CAD build for the part. Positions are in the model's coordinates, mm. A direction names the side the tool comes from. Round coordinates to 2 decimals unless told otherwise and drop trailing zeros. Order: outer loops, then holes, each group sorted by start corner. A loop starts at its lowest first (then second) coordinate and runs counter-clockwise, first axis right, second up. Notation, with made-up numbers: (81.5, 80.5) - (107.5, 80.5) arc R7 ccw to (107.5, 91.5) - close; hole circle Ø1 at (-35.75, 0.5). An arc over 180 degrees is marked (long way). Use one line per item in the form item = value. Start each with the question number.
from build123d import *

# Parameters (mm, degrees)
SKETCH1_W           = 60.96
SKETCH1_H           = 40.64
BOSS_EXTRUDE1_DEPTH = 5.08
SHELL1_T            = -2.54
SKETCH2_R           = 2.54
BOSS_EXTRUDE2_DEPTH = 5.08
SKETCH3_R           = 1.016
CUT_EXTRUDE1_DEPTH  = 5.08
FILLET2_R           = 1.27


with BuildPart() as part:
    # Sketch1 → Boss-Extrude1 (new body)
    with BuildSketch(Plane(origin=(0, 0, 0), x_dir=(1, 0, 0), z_dir=(0, 1, 0))):
        with Locations((30.48, 20.32)):
            Rectangle(SKETCH1_W, SKETCH1_H)
    extrude(amount=BOSS_EXTRUDE1_DEPTH)

    # Shell1
    shell1_openings = [part.faces().sort_by_distance(p)[0] for p in [
        (30.48, 0, -20.32),
    ]]
    offset(amount=SHELL1_T, openings=shell1_openings, kind=Kind.INTERSECTION)

    # Sketch2 → Boss-Extrude2 (add)
    with BuildSketch(Plane.XZ):
        with Locations((58.42, -38.1)):
            Circle(SKETCH2_R)
        with Locations((58.42, -2.54)):
            Circle(SKETCH2_R)
        with Locations((2.54, -2.54)):
            Circle(SKETCH2_R)
        with Locations((2.54, -38.1)):
            Circle(SKETCH2_R)
    extrude(amount=-BOSS_EXTRUDE2_DEPTH)

    # Sketch3 → Cut-Extrude1 (cut)
    with BuildSketch(Plane.XZ):
        with Locations((58.42, -38.1)):
            Circle(SKETCH3_R)
        with Locations((58.42, -2.54)):
            Circle(SKETCH3_R)
        with Locations((2.54, -2.54)):
            Circle(SKETCH3_R)
        with Locations((2.54, -38.1)):
            Circle(SKETCH3_R)
    extrude(amount=-CUT_EXTRUDE1_DEPTH, mode=Mode.SUBTRACT)

    # Fillet2
    fillet2_edges = [part.edges().sort_by_distance(p)[0] for p in [
        (60.96, 5.08, -20.32),
        (30.48, 5.08, -40.64),
        (0, 5.08, -20.32),
        (30.48, 5.08, 0),
        (0, 2.54, -40.64),
        (60.96, 2.54, -40.64),
        (60.96, 2.54, 0),
        (0, 2.54, 0),
    ]]
    fillet(fillet2_edges, radius=FILLET2_R)


solid = part.part
(1) Mould opens along X. For faces 1 (the flat face through (30, 2.54, -21)), 2 (the cylindrical face through (0.382, 4.718, -20.053)), 3 (the cylindrical face through (30.071, 4.718, -40.258)) say: pulls with the +X half, pulls with the -X half, needs draft (parallel to the pull), parting line crosses it, or undercut.
(2) Slice it at B-B (y = 1.5). Give the cut face in (x, z).
(3) Slice it at A-A (z = -6). Give the cut face in (x, y), and give its area (3 significant figures).
(4) Flat gauge pins, fed straight in: P1, Ø1.5, axis at x = 12.5, z = -30.5, coming from the -Y side; P2, Ø1.8, axis at x = 58.42, z = -38.1, coming from the -Y side. Where does each tip first touch, or does it go through?
(5) Slice it at C-C (x = 11.5). Give the cut face in (y, z).
(6) Which spindle directions (+Z, -Z, +X, -X, +Y, -Y) get a long thin tool onto all of the face, cutting with end or side? Do faces 4 (the flat face through (2.54, 1, -20)), 5 (the cylindrical face through (60.578, 1.932, -40.278)). Say none if no direction does.
(7) Wall check: line 1 (Z direction, x = 2.54, y = 3.45); line 2 (X direction, y = 2.5, z = -24.5); line 3 (Y direction, x = 36, z = -31). Give the ranges that are in metal, low to high. Write a range as [from, to].
Results list:
q1.face_1 = undercut
q1.face_2 = pulls with the -X half
q1.face_3 = needs draft
q2.outline = (0, -39.37) arc R1.27 ccw to (1.27, -40.64) - (59.69, -40.64) arc R1.27 ccw to (60.96, -39.37) - (60.96, -1.27) arc R1.27 ccw to (59.69, 0) - (1.27, 0) arc R1.27 ccw to (0, -1.27) - close; hole circle Ø2.03 at (2.54, -38.1); hole circle Ø2.03 at (2.54, -2.54); hole (2.54, -35.56) arc R2.54 cw to (5.08, -38.1) - (55.88, -38.1) arc R2.54 cw to (58.42, -35.56) - (58.42, -5.08) arc R2.54 cw to (55.88, -2.54) - (5.08, -2.54) arc R2.54 cw to (2.54, -5.08) - close; hole circle Ø2.03 at (58.42, -38.1); hole circle Ø2.03 at (58.42, -2.54)
q3.outline = (0, 0) - (2.54, 0) - (2.54, 2.54) - (58.42, 2.54) - (58.42, 0) - (60.96, 0) - (60.96, 3.81) arc R1.27 ccw to (59.69, 5.08) - (1.27, 5.08) arc R1.27 ccw to (0, 3.81) - close
q3.area = 167 mm²
q4.P1 = 2.54
q4.P2 = through
q5.outline = (0, -40.64) - (3.81, -40.64) arc R1.27 ccw to (5.08, -39.37) - (5.08, -1.27) arc R1.27 ccw to (3.81, 0) - (0, 0) - (0, -2.54) - (2.54, -2.54) - (2.54, -38.1) - (0, -38.1) - close
q6.face_4 = -Y
q6.face_5 = -Z, +X, +Y, -Y
q7.line_1 = [-40.64, -39.12], [-37.08, -3.56], [-1.52, 0]
q7.line_2 = [0, 2.54], [58.42, 60.96]
q7.line_3 = [2.54, 5.08]
